from build123d import *

# Parameters (mm, degrees)
SKETCH1_W                                            = 60
SKETCH1_H                                            = 50
BOSS_EXTRUDE1_DEPTH                                  = 6
CSK_FOR_M5_COUNTERSUNK_RAISED_HEAD_SCREW_D           = 5.3
CSK_FOR_M5_COUNTERSUNK_RAISED_HEAD_SCREW_CSINK_D     = 10.4
CSK_FOR_M5_COUNTERSUNK_RAISED_HEAD_SCREW_CSINK_ANGLE = 90
BOSS_EXTRUDE2_DEPTH                                  = 6
SKETCH6_R                                            = 3
CUT_EXTRUDE1_DEPTH                                   = 6


with BuildPart() as part:
    # Sketch1 → Boss-Extrude1 (new body)
    with BuildSketch(Plane(origin=(0, 0, 0), x_dir=(1, 0, 0), z_dir=(0, 1, 0))):
        Rectangle(SKETCH1_W, SKETCH1_H)
    extrude(amount=BOSS_EXTRUDE1_DEPTH)

    # CSK for M5 Countersunk Raised Head Screw1 (through all)
    with Locations(Plane(origin=(0, 6, 0), x_dir=(1, 0, 0), z_dir=(0, 1, 0))):
        with Locations((-20, -15), (16, -15), (16, 15), (-20, 15)):
            CounterSinkHole(CSK_FOR_M5_COUNTERSUNK_RAISED_HEAD_SCREW_D / 2, CSK_FOR_M5_COUNTERSUNK_RAISED_HEAD_SCREW_CSINK_D / 2, counter_sink_angle=CSK_FOR_M5_COUNTERSUNK_RAISED_HEAD_SCREW_CSINK_ANGLE)

    # Sketch5 → Boss-Extrude2 (add)
    with BuildSketch(Plane(origin=(30, 0, 0), x_dir=(0, 0, -1), z_dir=(1, 0, 0))):
        with BuildLine():
            Line((-25, 6), (-8.94427191, 38.11145618))
            ThreePointArc((-8.94427191, 38.11145618), (0, 43.639320225), (8.94427191, 38.11145618))
            Line((8.94427191, 38.11145618), (25, 6))
            Line((25, 6), (25, 0))
            Line((25, 0), (-25, 0))
            Line((-25, 0), (-25, 6))
        make_face()
    extrude(amount=BOSS_EXTRUDE2_DEPTH)

    # Sketch6 → Cut-Extrude1 (cut)
    with BuildSketch(Plane(origin=(36, 0, 0), x_dir=(0, 0, -1), z_dir=(1, 0, 0))):
        with Locations((0, 33.639320225)):
            Circle(SKETCH6_R)
    extrude(amount=-CUT_EXTRUDE1_DEPTH, mode=Mode.SUBTRACT)


solid = part.part
For this review, take the finished solid that the model builds, in its own axes (mm). A direction names the side the tool comes from. Round coordinates to 2 decimals unless told otherwise and drop trailing zeros. Loops run counter-clockwise (first coordinate to the right, second up) from the corner with the lowest first, then second, coordinate; pieces in that order, holes last. Notation, with made-up numbers: (-17, 79.25) - (38, 79.25) arc R28 cw to (38, 111.25) - close; hole circle Ø8 at (36, -28.75). An arc over 180 degrees is marked (long way). Use one line per item in the form item = value.
Item 1: Mouldability with a two-part tool opening along X and no side actions: class faces 1 (the conical face through (-19.639, 3.574, -17.75)), 2 (the flat face through (30, 21, 0)), 3 (the cylindrical face through (33.042, 36.614, 0.391)) as +X half, -X half, draft (parallel to the pull), parting line (faces both ways), or undercut.
Answers:
face_1 = undercut
face_2 = -X half
face_3 = draft
Item 2: Consider section B-B on x = 16. Write out the cut boundary in (y, z), then the cut area to 3 significant figures.
Answers:
outline = (0, -25) - (6, -25) - (6, -20.2) - (3.45, -17.65) - (0, -17.65) - close; (0, -12.35) - (3.45, -12.35) - (6, -9.8) - (6, 9.8) - (3.45, 12.35) - (0, 12.35) - close; (0, 17.65) - (3.45, 17.65) - (6, 20.2) - (6, 25) - (0, 25) - close
area = 223 mm^2
Item 3: Consider section D-D on y = 24.5. Write out the cut boundary in (x, z).
Answers:
outline = (30, -15.75) - (36, -15.75) - (36, 15.75) - (30, 15.75) - close
Item 4: Clearance check with flat-ended pins moving along their axes: P1, Ø7, axis at x = 16, z = -15, coming from the -Y side; P2, Ø1.5, axis at y = 34.5, z = 10.5, coming from the -X side; P3, Ø7, axis at x = 16, z = 15, coming from the +Y side; P4, Ø1.5, axis at x = -3.5, z = -3, coming from the +Y side. State where each tip first meets the part, or that it passes through.
Answers:
P1 = 0
P2 = 30
P3 = 4.3
P4 = 6
Item 5: For line 1 (X direction, y = 0.9, z = 15); line 2 (Z direction, x = 16, y = 0.85); line 3 (X direction, y = 17, z = 4.5), list the stretches that pass through material, from the lowest coordinate up.
Answers:
line_1 = -30 to -22.65, -17.35 to 13.35, 18.65 to 36
line_2 = -25 to -17.65, -12.35 to 12.35, 17.65 to 25
line_3 = 30 to 36
Item 6: Consider section C-C on z = 15. Write out the cut boundary in (x, y), then the cut area to 3 significant figures.
Answers:
outline = (-30, 0) - (-22.65, 0) - (-22.65, 3.45) - (-25.2, 6) - (-30, 6) - close; (-17.35, 0) - (13.35, 0) - (13.35, 3.45) - (10.8, 6) - (-14.8, 6) - (-17.35, 3.45) - close; (18.65, 0) - (36, 0) - (36, 26) - (30, 26) - (30, 6) - (21.2, 6) - (18.65, 3.45) - close
area = 439 mm^2
Item 7: Tool access review of faces 4 (the flat face through (0, 6, 0)), 5 (the flat face through (33, 22, 17)): name each direction out of +Z, -Z, +X, -X, +Y, -Y from which nothing blocks a thin tool from reaching the whole face with its end or side.
Answers:
face_4 = +Z, -Z, -X, +Y
face_5 = +Z, +X, -X, +Y
Item 8: Consider section A-A on z = 0. Write out the cut boundary in (x, y).
Answers:
outline = (-30, 0) - (36, 0) - (36, 30.64) - (30, 30.64) - (30, 6) - (-30, 6) - close; (30, 36.64) - (36, 36.64) - (36, 43.64) - (30, 43.64) - close
